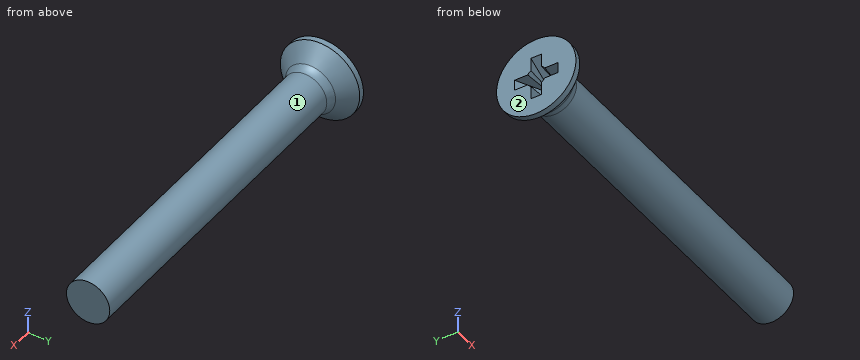
```python
from build123d import *

# Parameters (mm, degrees)
FILLET1_R    = 0.8
SKETCH3_W    = 0.74
SKETCH3_H    = 3
SKETCH4_W    = 0.74
SKETCH4_H    = 0.995702004
RECPAT_COUNT = 2
RECPAT_ANGLE = 90


with BuildPart() as part:
    # BodySke → Base-Revolve (revolve)
    with BuildSketch(Plane.XY):
        Polygon((0, 0), (0, 2.75), (0.4, 2.75), (1.65, 1.5), (25, 1.5), (25, 0), align=None)
    revolve(axis=Axis((-6.35, 0, 0), (1, 0, 0)))

    # Fillet1
    fillet1_edges = [part.edges().sort_by_distance(p)[0] for p in [
        (1.65, -1.5, 0),
    ]]
    fillet(fillet1_edges, radius=FILLET1_R)

    # Sketch3 → Recess section 0
    with BuildSketch(Plane.ZY):
        Rectangle(SKETCH3_W, SKETCH3_H)
    # Sketch4 → Recess section 1
    with BuildSketch(Plane.ZY.offset(-2.01)):
        Rectangle(SKETCH4_W, SKETCH4_H)
    recess = loft(mode=Mode.SUBTRACT)

    # RecPat: Recess ×2 about axis
    recpat_axis = Axis((0, 0, 0), (1, 0, 0))
    for i in range(1, RECPAT_COUNT):
        add(recess.rotate(recpat_axis, i * RECPAT_ANGLE / (RECPAT_COUNT - 1)), mode=Mode.SUBTRACT)

    # RecCorSke → RecessCore (revolve, cut)
    with BuildSketch(Plane.XY):
        Polygon((0, 0), (0, 0.696552892), (2.01, 0.556), (2.190655351, 0), align=None)
    revolve(axis=Axis((-3.175, 0, 0), (1, 0, 0)), mode=Mode.SUBTRACT)


solid = part.part
```
Model file for the job. Use its own axes, mm. Face numbers are marked on the shaded views. A direction names the side the tool comes from. Give positions to 0.01 mm unless a question says otherwise; leave off trailing zeros. Order: outer loops, then holes, each group sorted by start corner. A loop starts at its lowest first (then second) coordinate and runs counter-clockwise, first axis right, second up.
1) Saw through at A-A, the plane x = 12.25. Write the cut outline in (y, z).
2) 3-axis set-ups, long thin cutter, end or side, ignore diameter. For the marked faces 1 and 2: which of +Z, -Z, +X, -X, +Y, -Y reach the whole face in a straight line?
3) Wall check: probe 1 along X at (y, z) = (-1.2, 1.15); probe 2 along Y at (x, z) = (19.5, -0.1); probe 3 along Z at (x, y) = (4.25, 0.4). Give the ranges that are in metal, low to high.
4) Pin check, flat tips, straight feed: pin 1 (3 mm diameter, centred on x = 5, y = 1, fed in from -Z); pin 2 (3 mm diameter, centred on x = 21, z = 1.5, fed in from +Y). Stop position of each tip, or through.
Computed:
1. outline: circle Ø3 at (0, 0)
2. face 1: +X
2. face 2: +Z, -Z, -X, +Y, -Y
3. probe 1: x = 0 to 1.5
3. probe 2: y = -1.5 to 1.5
3. probe 3: z = -1.45 to 1.45
4. pin 1: stops at z = -1.5
4. pin 2: stops at y = 1.5
